```python
from build123d import *

# Parameters (mm, degrees)
SKETCH1_W                                        = 61
SKETCH1_H                                        = 6.1
BOSS_EXTRUDE1_DEPTH                              = 22.5
SKETCH2_OUTSIDE_W                                = 76.06
SKETCH2_OUTSIDE_H                                = 21.16
SKETCH2_OUTSIDE_W_2                              = 61
SKETCH2_OUTSIDE_H_2                              = 5.41284
CUT_EXTRUDE1_DEPTH                               = 6
CUT_EXTRUDE3_DEPTH                               = 23.5
SKETCH6_R                                        = 3.175
CUT_EXTRUDE4_DEPTH                               = 7.1
SKETCH7_R                                        = 1.5
CUT_EXTRUDE5_DEPTH                               = 7.1
M2_5X0_45_TAPPED_HOLE1_D                         = 2.05
M2_5X0_45_TAPPED_HOLE2_D                         = 2.05
M2_5X0_45_TAPPED_HOLE2_DEPTH                     = 7.3
M2_5X0_45_TAPPED_HOLE2_TIP                       = 0.615882135
CBORE_FOR_M3_PAN_HEAD_MACHINE_SCREW1_D           = 3.4
CBORE_FOR_M3_PAN_HEAD_MACHINE_SCREW1_CBORE_D     = 6.5
CBORE_FOR_M3_PAN_HEAD_MACHINE_SCREW1_CBORE_DEPTH = 2.2


with BuildPart() as part:
    # Sketch1 → Boss-Extrude1 (new body)
    with BuildSketch(Plane(origin=(0, 0, 0), x_dir=(0, 0, -1), z_dir=(1, 0, 0))):
        with Locations((30.5, 0)):
            Rectangle(SKETCH1_W, SKETCH1_H)
    extrude(amount=BOSS_EXTRUDE1_DEPTH)

    # Sketch2 outside → Cut-Extrude1 (cut)
    with BuildSketch(Plane(origin=(22.5, 0, 0), x_dir=(0, 0, -1), z_dir=(1, 0, 0))):
        with Locations((30.5, 0)):
            Rectangle(SKETCH2_OUTSIDE_W, SKETCH2_OUTSIDE_H)
        with Locations((30.5, 0)):
            Rectangle(SKETCH2_OUTSIDE_W_2, SKETCH2_OUTSIDE_H_2, mode=Mode.SUBTRACT)
    extrude(amount=-CUT_EXTRUDE1_DEPTH, mode=Mode.SUBTRACT)

    # Sketch5 → Cut-Extrude3 (cut, through all)
    with BuildSketch(Plane.ZY):
        with BuildLine():
            Line((-43.5866, -0.01898), (-43.5866, -3.05))
            Line((-43.5866, -3.05), (-48.6514, -3.05))
            Line((-48.6514, -3.05), (-48.6514, -0.01898))
            ThreePointArc((-48.6514, -0.01898), (-46.119, 2.51342), (-43.5866, -0.01898))
        make_face()
    extrude(amount=-CUT_EXTRUDE3_DEPTH, mode=Mode.SUBTRACT)

    # Sketch6 → Cut-Extrude4 (cut, through all)
    with BuildSketch(Plane(origin=(0, 3.05, 0), x_dir=(1, 0, 0), z_dir=(0, 1, 0))):
        with Locations(Location((7.5, 30.5, 0), (0, 0, 270))):  # turned: the seam where the file's is
            Circle(SKETCH6_R)
    extrude(amount=-CUT_EXTRUDE4_DEPTH, mode=Mode.SUBTRACT)

    # Sketch7 → Cut-Extrude5 (cut, through all)
    with BuildSketch(Plane(origin=(0, 3.05, 0), x_dir=(1, 0, 0), z_dir=(0, 1, 0))):
        with Locations(Location((5, 55.5, 0), (0, 0, 270))):  # turned: the seam where the file's is
            Circle(SKETCH7_R)
        with Locations(Location((5, 5.5, 0), (0, 0, 270))):  # turned: the seam where the file's is
            Circle(SKETCH7_R)
    extrude(amount=-CUT_EXTRUDE5_DEPTH, mode=Mode.SUBTRACT)

    # M2.5x0.45 Tapped Hole1 (through all)
    with Locations(Plane(origin=(0, -3.05, 0), x_dir=(-1, 0, 0), z_dir=(0, -1, 0))):
        with Locations((-5, 18)):
            Hole(M2_5X0_45_TAPPED_HOLE1_D / 2)

    # M2.5x0.45 Tapped Hole2
    with Locations(Plane(origin=(0, 0, -61), x_dir=(-1, 0, 0), z_dir=(0, 0, -1))):
        with Locations((-10, 0)):
            Hole(M2_5X0_45_TAPPED_HOLE2_D / 2, depth=M2_5X0_45_TAPPED_HOLE2_DEPTH)
            with Locations((0, 0, -(M2_5X0_45_TAPPED_HOLE2_DEPTH + M2_5X0_45_TAPPED_HOLE2_TIP / 2))):  # 118° drill point
                Cone(0, M2_5X0_45_TAPPED_HOLE2_D / 2, M2_5X0_45_TAPPED_HOLE2_TIP, mode=Mode.SUBTRACT)

    # CBORE for M3 Pan Head Machine Screw1 (through all)
    with Locations(Plane(origin=(0, -3.05, 0), x_dir=(-1, 0, 0), z_dir=(0, -1, 0))):
        with Locations((-11, 54.825), (-11, 17.15)):
            CounterBoreHole(CBORE_FOR_M3_PAN_HEAD_MACHINE_SCREW1_D / 2, CBORE_FOR_M3_PAN_HEAD_MACHINE_SCREW1_CBORE_D / 2, CBORE_FOR_M3_PAN_HEAD_MACHINE_SCREW1_CBORE_DEPTH)


solid = part.part
```
Source: CAD feature listing. Evaluate the final solid. Frame: model axes, mm. A direction names the side the tool comes from. Give positions to 0.01 mm unless a question says otherwise; leave off trailing zeros. Loops run counter-clockwise (first coordinate to the right, second up) from the corner with the lowest first, then second, coordinate; pieces in that order, holes last. Notation, with made-up numbers: (13, 52) - (56, 52) arc R25 ccw to (56, 81) - close; hole circle Ø6 at (2.5, 68). An arc over 180 degrees is marked (long way). Use CSV: the item, a comma, the result in double quotes.
1) Cut plane B-B (y = -1.75). Output: boundary loops of the cut face in (x, z) (3 decimals), and give its area (3 significant figures).
Worked out:
outline,"(0, -61) - (22.5, -61) - (22.5, -48.651) - (0, -48.651) - close; (0, -43.587) - (22.5, -43.587) - (22.5, 0) - (0, 0) - close; hole circle Ø3 at (5, -55.5); hole circle Ø3 at (5, -5.5); hole circle Ø2.05 at (5, -18); hole circle Ø6.35 at (7.5, -30.5); hole circle Ø6.5 at (11, -54.825); hole circle Ø6.5 at (11, -17.15)"
area,"1,140 mm^2"
2) Set-up query: faces 5 (the flat face through (10, -0.85, -53)), 6 (the flat face through (20, 2.706, -30)), 7 (the flat face through (20, -2.706, -55)). Return all of +Z, -Z, +X, -X, +Y, -Y with unobstructed straight access to the full face (end or side cutting, diameter ignored); none if empty.
Worked out:
face 5,"-Y"
face 6,"+Z, -Z, +X, +Y"
face 7,"+Z, -Z, +X, -Y"
3) Mould query, pull axis X, two halves, no side actions, for faces 1 (the flat face through (0, 0, -30)), 2 (the cylindrical face through (4.867, 0.043, -19.016)), 3 (the flat face through (8, -3.05, -21)), 4 (the cylindrical face through (5, 0, -7)). Classes: +X half, -X half, draft (parallel to the pull), parting line (faces both ways), or undercut.
Worked out:
face 1,"-X half"
face 2,"undercut"
face 3,"draft"
face 4,"undercut"
4) Cut plane A-A (z = -5.5). Output: boundary loops of the cut face in (x, y), and give its area (3 significant figures).
Worked out:
outline,"(0, -3.05) - (3.5, -3.05) - (3.5, 3.05) - (0, 3.05) - close; (6.5, -3.05) - (16.5, -3.05) - (16.5, -2.71) - (22.5, -2.71) - (22.5, 2.71) - (16.5, 2.71) - (16.5, 3.05) - (6.5, 3.05) - close"
area,"115 mm^2"
5) Cut plane D-D (z = -18). Output: boundary loops of the cut face in (x, y) (3 decimals), and give its area (3 significant figures).
Worked out:
outline,"(0, -3.05) - (3.975, -3.05) - (3.975, 3.05) - (0, 3.05) - close; (6.025, -3.05) - (7.863, -3.05) - (7.863, -0.85) - (9.528, -0.85) - (9.528, 3.05) - (6.025, 3.05) - close; (12.472, -0.85) - (14.137, -0.85) - (14.137, -3.05) - (16.5, -3.05) - (16.5, -2.706) - (22.5, -2.706) - (22.5, 2.706) - (16.5, 2.706) - (16.5, 3.05) - (12.472, 3.05) - close"
area,"95.3 mm^2"
6) Cut plane C-C (x = 5). Output: boundary loops of the cut face in (y, z) (3 decimals), and give its area (3 significant figures).
Worked out:
outline,"(-3.05, -61) - (3.05, -61) - (3.05, -57) - (-3.05, -57) - close; (-3.05, -54) - (3.05, -54) - (3.05, -32.457) - (-3.05, -32.457) - (-3.05, -43.587) - (-0.019, -43.587) arc R2.532 cw to (-0.019, -48.651) - (-3.05, -48.651) - close; (-3.05, -28.543) - (3.05, -28.543) - (3.05, -19.025) - (-3.05, -19.025) - close; (-3.05, -16.975) - (3.05, -16.975) - (3.05, -7) - (-3.05, -7) - close; (-3.05, -4) - (3.05, -4) - (3.05, 0) - (-3.05, 0) - close"
area,"274 mm^2"
7) Pin query (flat end, axial travel): P1, Ø1.8, axis at x = 20, z = -56, coming from the -Y side; P2, Ø4, axis at x = 11, z = -17.15, coming from the -Y side; P3, Ø1.8, axis at x = 5, z = -5.5, coming from the +Y side. Return the tip coordinate at first contact, or that it passes through.
Worked out:
P1,"stops at y = -2.71"
P2,"stops at y = -0.85"
P3,"passes through"
8) Line query: line 1 (X direction, y = -2.2, z = -17.15); line 2 (X direction, y = -1.25, z = -56.5); line 3 (Z direction, x = 16.5, y = -2.5). Output: solid intervals per line, ascending.
Worked out:
line 1,"x = 0 to 4.43, 5.57 to 7.75, 14.25 to 22.5"
line 2,"x = 0 to 3.88, 6.12 to 8.21, 13.79 to 22.5"
line 3,"z = -61 to -48.65, -43.59 to 0"
